Source: CAD feature listing. Evaluate the final solid. Frame: model axes, mm. A direction names the side the tool comes from. Round coordinates to 2 decimals unless told otherwise and drop trailing zeros. Write each loop counter-clockwise with the first axis right and the second up, starting at its lowest first coordinate (ties: lowest second). Pieces come first, ordered by that corner, then holes.
```python
from build123d import *

# Parameters (mm, degrees)
SKETCH1_W           = 127.762
SKETCH1_H           = 85.598
SKETCH1_W_2         = 122.936
SKETCH1_H_2         = 80.772
BOSS_EXTRUDE1_DEPTH = 3.048
SKETCH2_W           = 122.936
SKETCH2_H           = 80.772
BOSS_EXTRUDE2_DEPTH = 2.413
SKETCH3_W           = 122.936
SKETCH3_H           = 80.772
SKETCH3_W_2         = 116.332
SKETCH3_H_2         = 77.978
SKETCH3_W_3         = 1.524
BOSS_EXTRUDE3_DEPTH = 11.43


with BuildPart() as part:
    # Sketch1 → Boss-Extrude1 (new body)
    with BuildSketch(Plane(origin=(0, 0, 0), x_dir=(1, 0, 0), z_dir=(0, 1, 0))):
        with Locations((63.881, -42.799)):
            Rectangle(SKETCH1_W, SKETCH1_H)
        with Locations((63.881, -42.799)):
            Rectangle(SKETCH1_W_2, SKETCH1_H_2, mode=Mode.SUBTRACT)
    extrude(amount=BOSS_EXTRUDE1_DEPTH)

    # Sketch2 → Boss-Extrude2 (add)
    with BuildSketch(Plane(origin=(0, 3.048, 0), x_dir=(1, 0, 0), z_dir=(0, 1, 0))):
        with Locations((63.881, -42.799)):
            Rectangle(SKETCH2_W, SKETCH2_H)
    extrude(amount=-BOSS_EXTRUDE2_DEPTH)

    # Sketch3 → Boss-Extrude3 (add)
    with BuildSketch(Plane(origin=(0, 3.048, 0), x_dir=(1, 0, 0), z_dir=(0, 1, 0))):
        with Locations((63.881, -42.799)):
            Rectangle(SKETCH3_W, SKETCH3_H)
        with Locations((63.881, -42.799)):
            Rectangle(SKETCH3_W_2, SKETCH3_H_2, mode=Mode.SUBTRACT)
        with Locations((34.417, -42.799)):
            Rectangle(SKETCH3_W_3, SKETCH3_H_2)
        with Locations((63.881, -42.799)):
            Rectangle(SKETCH3_W_3, SKETCH3_H_2)
        with Locations((93.345, -42.799)):
            Rectangle(SKETCH3_W_3, SKETCH3_H_2)
    extrude(amount=BOSS_EXTRUDE3_DEPTH)


solid = part.part
```
Q1. Pin query (flat end, axial travel): P1, Ø1, axis at y = 4.5, z = 16, coming from the -X side; P2, Ø5.5, axis at y = 8, z = 46, coming from the +X side; P3, Ø1.5, axis at x = 86, z = 55.5, coming from the +Y side. Return the tip coordinate at first contact, or that it passes through.
Q2. Section query B-B, the plane x = 42.5. Output: boundary loops of the cut face in (y, z) (3 decimals).
Q3. Mould query, pull axis X, two halves, no side actions, for faces 4 (the face through (63, 9, 83.185)), 5 (the face through (64.643, 9, 43)), 6 (the face through (122.047, 9, 43)), 7 (the face through (2.413, 9, 43)). Classes: pulls with the +X half, pulls with the -X half, needs draft (parallel to the pull), parting line crosses it, or undercut.
Q4. Line query: line 1 (X direction, y = 14.25, z = 30) (3 decimals); line 2 (Z direction, x = 39, y = 8.5) (3 decimals); line 3 (Y direction, x = 37, z = 72) (3 decimals). Output: solid intervals per line, ascending.
Q5. Section query A-A, the plane y = 9. Output: boundary loops of the cut face in (x, z) (3 decimals).
Q6. Section query C-C, the plane z = 70. Output: boundary loops of the cut face in (x, y) (3 decimals), and give its area (3 significant figures).
Q7. Set-up query: faces 1 (the face through (63, 2, 0)), 2 (the face through (63, 9, 2.413)), 3 (the face through (19, 3.048, 42)). Return all of +Z, -Z, +X, -X, +Y, -Y with unobstructed straight access to the full face (end or side cutting, diameter ignored); none if empty.
Filled in:
1. P1: stops at x = 2.41
1. P2: stops at x = 125.35
1. P3: stops at y = 3.05
2. outline: (0, 0) - (3.048, 0) - (3.048, 2.413) - (14.478, 2.413) - (14.478, 3.81) - (3.048, 3.81) - (3.048, 81.788) - (14.478, 81.788) - (14.478, 83.185) - (3.048, 83.185) - (3.048, 85.598) - (0, 85.598) - (0, 83.185) - (0.635, 83.185) - (0.635, 2.413) - (0, 2.413) - close
3. face 4: needs draft
3. face 5: undercut
3. face 6: undercut
3. face 7: pulls with the -X half
4. line 1: x = 2.413 to 5.715, 33.655 to 35.179, 63.119 to 64.643, 92.583 to 94.107, 122.047 to 125.349
4. line 2: z = 2.413 to 3.81, 81.788 to 83.185
4. line 3: y = 0.635 to 3.048
5. outline: (2.413, 2.413) - (125.349, 2.413) - (125.349, 83.185) - (2.413, 83.185) - close; hole (5.715, 3.81) - (33.655, 3.81) - (33.655, 81.788) - (5.715, 81.788) - close; hole (35.179, 3.81) - (63.119, 3.81) - (63.119, 81.788) - (35.179, 81.788) - close; hole (64.643, 3.81) - (92.583, 3.81) - (92.583, 81.788) - (64.643, 81.788) - close; hole (94.107, 3.81) - (122.047, 3.81) - (122.047, 81.788) - (94.107, 81.788) - close
6. outline: (0, 0) - (2.413, 0) - (2.413, 0.635) - (125.349, 0.635) - (125.349, 0) - (127.762, 0) - (127.762, 3.048) - (125.349, 3.048) - (125.349, 14.478) - (122.047, 14.478) - (122.047, 3.048) - (94.107, 3.048) - (94.107, 14.478) - (92.583, 14.478) - (92.583, 3.048) - (64.643, 3.048) - (64.643, 14.478) - (63.119, 14.478) - (63.119, 3.048) - (35.179, 3.048) - (35.179, 14.478) - (33.655, 14.478) - (33.655, 3.048) - (5.715, 3.048) - (5.715, 14.478) - (2.413, 14.478) - (2.413, 3.048) - (0, 3.048) - close
6. area: 439 mm2
7. face 1: -Z, +X, -X, +Y, -Y
7. face 2: -Z, +X, -X, +Y
7. face 3: +Y
